Part model, mm, in its own coordinate system. Round coordinates to 2 decimals unless told otherwise and drop trailing zeros. Write each loop counter-clockwise with the first axis right and the second up, starting at its lowest first coordinate (ties: lowest second). Pieces come first, ordered by that corner, then holes. Notation, with made-up numbers: M -38,11.5 L 15,11.5 A27 ccw 15,28.5 Z; hole C 53.25,84.25 d3. An arc over 180 degrees is marked long. Answer as a JSON object with one key per item and string values. Group by question number.
1. Band-saw the part on A-A, the plane x = 0. Write the cut outline in (y, z) (3 decimals).
2. Drop flat-ended pins along their axis: pin 1 (2 mm diameter, centred on y = -4.5, z = 3.5, fed in from -X); pin 2 (1 mm diameter, centred on y = -122, z = 3.5, fed in from -X); pin 3 (1.6 mm diameter, centred on x = 0.5, z = 3.5, fed in from +Y); pin 4 (2 mm diameter, centred on y = -120, z = 4, fed in from +X). Give the stop position or say it passes through.
3. Drill centre lines: line 1 (Y direction, x = 0, z = 4.25) (3 decimals); line 2 (Z direction, x = -2.75, y = -98.5). Where is each one in solid material? Low to high. Write a range as from..to.
4. Band-saw the part on C-C, the plane z = 1.25. Write the cut outline in (x, y).
5. Band-saw the part on B-B, the plane y = -90. Write the cut outline in (x, z) (3 decimals), plus the area to 3 significant figures.
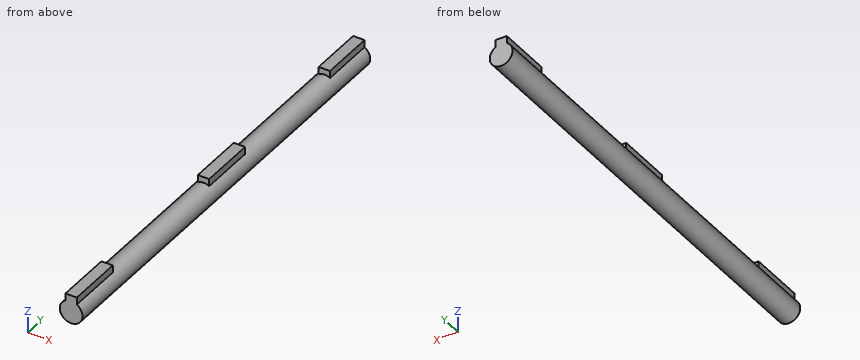
from build123d import *

# Parameters (mm, degrees)
F0_R     = 3.175
F1_DEPTH = 127
F2_W     = 1.5875
F2_H     = 3.175
F3_DEPTH = 15.875
F5_W     = 3.175
F5_H     = 3.175
F6_DEPTH = 15.875
F8_W     = 3.175
F8_H     = 3.1142037669
F9_DEPTH = 15.24


with BuildPart() as f1:
    # F0 (on Front) → F1 (new body)
    with BuildSketch(Plane.XZ):
        Circle(F0_R)
    extrude(amount=F1_DEPTH)

    # F2 (on face) → F3 (join)
    with BuildSketch(Plane.XZ.offset(127)):
        with Locations((-0.79375, 3.1877)):
            Rectangle(F2_W, F2_H)
        with Locations((0.79375, 3.1877)):
            Rectangle(F2_W, F2_H)
    extrude(amount=-F3_DEPTH)

    # F5 (on offset) → F6 (join)
    with BuildSketch(Plane.XZ.offset(68.58)):
        with Locations((0, 3.1877)):
            Rectangle(F5_W, F5_H)
    extrude(amount=-F6_DEPTH)

    # F8 (on offset) → F9 (join)
    with BuildSketch(Plane.XZ.offset(15.24)):
        with Locations((0, 3.2180981166)):
            Rectangle(F8_W, F8_H)
    extrude(amount=-F9_DEPTH)


solid = f1.part
Worked answers:
{
 "1": {"outline": "M -127,-3.175 L 0,-3.175 L 0,4.775 L -15.24,4.775 L -15.24,3.175 L -52.705,3.175 L -52.705,4.775 L -68.58,4.775 L -68.58,3.175 L -111.125,3.175 L -111.125,4.775 L -127,4.775 Z"},
 "2": {"pin 1": "stops at x = -1.96", "pin 2": "stops at x = -1.59", "pin 3": "stops at y = 0", "pin 4": "stops at x = 1.59"},
 "3": {"line 1": "y = -127..-111.125, -68.58..-52.705, -15.24..0", "line 2": "z = -1.59..1.59"},
 "4": {"outline": "M -2.92,-127 L 2.92,-127 L 2.92,0 L -2.92,0 Z"},
 "5": {"outline": "C 0,0 d6.35", "area": "31.7 mm^2"}
}
